Build history of the part. All positions in model axes, mm. A direction names the side the tool comes from. Coordinates: 2 decimals unless noted, no trailing zeros. Order: outer loops, then holes, each group sorted by start corner. A loop starts at its lowest first (then second) coordinate and runs counter-clockwise, first axis right, second up. Notation, with made-up numbers: M 17,67.25 L 68,67.25 A12 ccw 68,73.25 Z; hole C -40,-8 d3. An arc over 180 degrees is marked long. Use a Markdown table: item, result. Add a question column.
from build123d import *

# Parameters (mm, degrees)
SKETCH1_W           = 406.4
SKETCH1_H           = 25.4
BOSS_EXTRUDE1_DEPTH = 24.13
SKETCH3_R           = 2.57175
CUT_EXTRUDE1_DEPTH  = 39.624
BOSS_EXTRUDE2_DEPTH = 39.624


with BuildPart() as part:
    # Sketch1 → Boss-Extrude1 (new body)
    with BuildSketch(Plane.XY):
        with Locations((-203.2, -12.7)):
            Rectangle(SKETCH1_W, SKETCH1_H)
    extrude(amount=BOSS_EXTRUDE1_DEPTH)

    # Sketch3 → Cut-Extrude1 (cut)
    with BuildSketch(Plane.XY.offset(24.13)):
        with Locations((-379.949777658, 0)):
            Circle(SKETCH3_R)
        with Locations((-340.071777658, 0)):
            Circle(SKETCH3_R)
        with Locations((-300.193777658, 0)):
            Circle(SKETCH3_R)
        with Locations((-260.315777658, 0)):
            Circle(SKETCH3_R)
        with Locations((-220.437777658, 0)):
            Circle(SKETCH3_R)
        with Locations((-180.559777658, 0)):
            Circle(SKETCH3_R)
        with Locations((-140.681777658, 0)):
            Circle(SKETCH3_R)
        with Locations((-100.803777658, 0)):
            Circle(SKETCH3_R)
        with Locations((-60.925777658, 0)):
            Circle(SKETCH3_R)
        with Locations((-21.047777658, 0)):
            Circle(SKETCH3_R)
    extrude(amount=-CUT_EXTRUDE1_DEPTH, mode=Mode.SUBTRACT)

    # Sketch4 → Boss-Extrude2 (add)
    with BuildSketch(Plane.XY.offset(24.13)):
        Polygon((-377.378027658, 0), (-360.010777658, 5.08), (-342.643527658, 0), align=None)
        Polygon((-337.500027658, 0), (-320.132777658, 5.08), (-302.765527658, 0), align=None)
        Polygon((-297.622027658, 0), (-280.254777658, 5.08), (-262.887527658, 0), align=None)
        Polygon((-257.744027658, 0), (-240.376777658, 5.08), (-223.009527658, 0), align=None)
        Polygon((-217.866027658, 0), (-200.498777658, 5.08), (-183.131527658, 0), align=None)
        Polygon((-177.988027658, 0), (-160.620777658, 5.08), (-143.253527658, 0), align=None)
        Polygon((-138.110027658, 0), (-120.742777658, 5.08), (-103.375527658, 0), align=None)
        Polygon((-98.232027658, 0), (-80.864777658, 5.08), (-63.497527658, 0), align=None)
        Polygon((-58.354027658, 0), (-40.986777658, 5.08), (-23.619527658, 0), align=None)
    extrude(amount=-BOSS_EXTRUDE2_DEPTH)


solid = part.part
(1) Which spindle directions (+Z, -Z, +X, -X, +Y, -Y) get a long thin tool onto all of the face, cutting with end or side? Do faces 1 (the flat face through (-206, -25.4, 12)), 2 (the flat face through (-89.67, 2.504, 4.595)), 3 (the flat face through (-200, 0, -8)). Say none if no direction does.
(2) Mould opens along X. For faces 4 (the flat face through (-152.059, 2.576, 4.595)), 5 (the flat face through (-206, -13, 0)), 6 (the flat face through (-32.425, 2.576, 4.595)) say: released by +X, released by -X, zero draft, split by the parting line, or undercut.
(3) Drill centre lines: line 1 along Z through (x, y) = (-184.5, -9); line 2 along Y through (x, z) = (-300.5, 6.5); line 3 along Y through (x, z) = (-358, -12). Where is each one in solid material? Low to high. Write a range as from..to.
(4) Slice it at A-A on z = -6.5. State how many separate pieces and enclosed holes the cut face has, and give its area (3 significant figures).
(5) Slice it at D-D on x = -208. Give the cut face in (y, z), and give its area (3 significant figures).
(6) Slice it at C-C on y = -20. Give the cut face in (x, z).
(7) Drop flat-ended pins along their axis: P1, Ø7.5, axis at x = -152.5, y = -15, coming from the -Z side; P2, Ø12.5, axis at x = -161.5, z = -11, coming from the -Y side; P3, Ø19, axis at x = -395, z = 6.5, coming from the +Y side. Give the stop position or say it passes through.
Solutions:
| question | item | result |
|---|---|---|
| 1 | face 1 | +Z, -Z, +X, -X, -Y |
| 1 | face 2 | +Z, -Z, +Y |
| 1 | face 3 | -Z, +X, -X, -Y |
| 2 | face 4 | undercut |
| 2 | face 5 | zero draft |
| 2 | face 6 | released by +X |
| 3 | line 1 | 0..24.13 |
| 3 | line 2 | -25.4..-2.55 |
| 3 | line 3 | 0..4.49 |
| 4 | separate pieces | 9 |
| 4 | enclosed holes | 0 |
| 4 | area | 794 mm² |
| 5 | outline | M -25.4,0 L 0,0 L 0,-15.49 L 2.89,-15.49 L 2.89,24.13 L -25.4,24.13 Z |
| 5 | area | 727 mm² |
| 6 | outline | M -406.4,0 L 0,0 L 0,24.13 L -406.4,24.13 Z |
| 7 | P1 | z = 0 |
| 7 | P2 | y = 0 |
| 7 | P3 | y = 0 |
